Work out the finished part from the listing and answer in its coordinate system (mm). Face numbers are marked on the shaded views. A direction names the side the tool comes from. Coordinates: 2 decimals unless noted, no trailing zeros. Order: outer loops, then holes, each group sorted by start corner. A loop starts at its lowest first (then second) coordinate and runs counter-clockwise, first axis right, second up.
```python
from build123d import *

# Parameters (mm, degrees)
F0_W          = 57.15
F0_H          = 57.15
F0_W_2        = 51.054
F0_H_2        = 51.054
F1_DEPTH      = 200.66
F2_R          = 3.048
F3_R          = 6.35
F5_DEPTH      = 28.576
F5_DEPTH_BACK = 28.576


with BuildPart() as f1:
    # F0 (on Top) → F1 (new body)
    with BuildSketch(Plane.XY):
        Rectangle(F0_W, F0_H)
        Rectangle(F0_W_2, F0_H_2, mode=Mode.SUBTRACT)
    extrude(amount=F1_DEPTH)

    # F2
    f2_edges = [f1.edges().sort_by_distance(p)[0] for p in [
        (25.527, 25.527, 100.33),
        (-25.527, 25.527, 100.33),
        (-25.527, -25.527, 100.33),
        (25.527, -25.527, 100.33),
    ]]
    fillet(f2_edges, radius=F2_R)

    # F3
    f3_edges = [f1.edges().sort_by_distance(p)[0] for p in [
        (-28.575, 28.575, 100.33),
        (-28.575, -28.575, 100.33),
        (28.575, -28.575, 100.33),
        (28.575, 28.575, 100.33),
    ]]
    fillet(f3_edges, radius=F3_R)

    # F4 (on Front) → F5 (cut, two sides)
    with BuildSketch(Plane.XZ) as f5_sk:
        Polygon((-28.575, 200.66), (28.575, 143.51), (28.575, 200.66), align=None)
    extrude(amount=-F5_DEPTH, mode=Mode.SUBTRACT)
    extrude(f5_sk.sketch, amount=F5_DEPTH_BACK, mode=Mode.SUBTRACT)


solid = f1.part
```
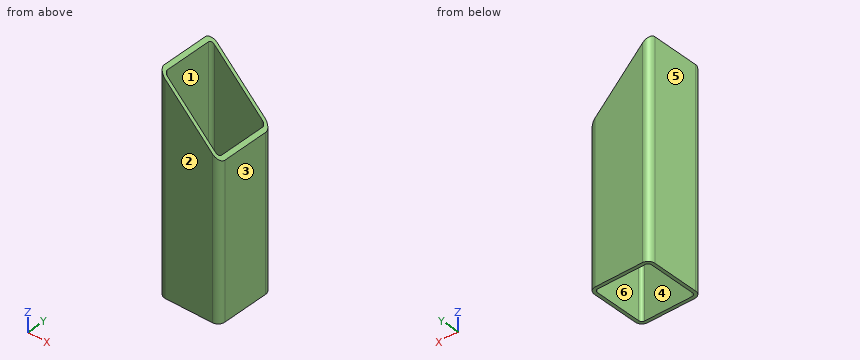
1. The part is cut by section D-D (z = 188). Determine the outline of the cut face in (x, y) (3 decimals).
2. The part is cut by section A-A (y = 13). Determine the outline of the cut face in (x, z) (3 decimals).
3. The part is cut by section C-C (x = -18). Determine the outline of the cut face in (y, z) (3 decimals), plus the area to 3 significant figures.
4. A flat-ended cylindrical pin translates along its axis: pin 1 (12 mm diameter, centred on x = -3.5, y = -14, fed in from -Z) (3 decimals). Find the tip coordinate at first contact, or state that the pin passes through.
5. The mould has two halves that part along Y. Classify the marked faces 1, 2, 3 and 4: released by +Y, released by -Y, zero draft, split by the parting line, or undercut.
6. The part is cut by section B-B (z = 92.5). Determine the outline of the cut face in (x, y) (3 decimals), plus the area to 3 significant figures.
7. For the marked faces 5 and 6, determine the directions among +Z, -Z, +X, -X, +Y, -Y from which every point of the face is accessible in a straight line to the end or side of a thin tool.
8. Consider probe 1 along Y at (x, z) = (22, 104.5) (3 decimals); probe 2 along X at (y, z) = (6, 165) (3 decimals). Determine where each line is inside the solid, lowest interval first.
Worked out:
1. outline: (-28.575, -22.225) arc R6.35 ccw to (-22.225, -28.575) - (-15.915, -28.575) - (-15.915, -25.527) - (-22.479, -25.527) arc R3.048 cw to (-25.527, -22.479) - (-25.527, 22.479) arc R3.048 cw to (-22.479, 25.527) - (-15.915, 25.527) - (-15.915, 28.575) - (-22.225, 28.575) arc R6.35 ccw to (-28.575, 22.225) - close
2. outline: (-28.575, 0) - (-25.527, 0) - (-25.527, 197.612) - (-28.575, 200.66) - close; (25.527, 0) - (28.575, 0) - (28.575, 143.51) - (25.527, 146.558) - close
3. outline: (-28.575, 0) - (-25.527, 0) - (-25.527, 190.085) - (-28.575, 190.085) - close; (25.527, 0) - (28.575, 0) - (28.575, 190.085) - (25.527, 190.085) - close
3. area: 1,160 mm2
4. pin 1: passes through
5. face 1: undercut
5. face 2: released by -Y
5. face 3: zero draft
5. face 4: undercut
6. outline: (-28.575, -22.225) arc R6.35 ccw to (-22.225, -28.575) - (22.225, -28.575) arc R6.35 ccw to (28.575, -22.225) - (28.575, 22.225) arc R6.35 ccw to (22.225, 28.575) - (-22.225, 28.575) arc R6.35 ccw to (-28.575, 22.225) - close; hole (-25.527, -22.479) arc R3.048 ccw to (-22.479, -25.527) - (22.479, -25.527) arc R3.048 ccw to (25.527, -22.479) - (25.527, 22.479) arc R3.048 ccw to (22.479, 25.527) - (-22.479, 25.527) arc R3.048 ccw to (-25.527, 22.479) - close
6. area: 633 mm2
7. face 5: +Z, -Z, -X, +Y, -Y
7. face 6: +Z, -Z
8. probe 1: y = -28.575 to -25.527, 25.527 to 28.575
8. probe 2: x = -28.575 to -25.527
